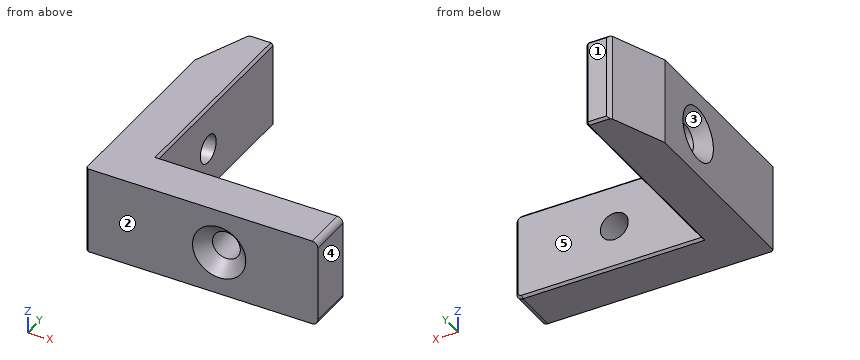
from build123d import *
from OCP.BRepFilletAPI import BRepFilletAPI_MakeChamfer

# Parameters (mm, degrees)
BOSS_EXTRUDE1_DEPTH                                  = 7.5
CSK_FOR_M4_HEX_SOCKET_COUNTERSUNK_HEAD_S_D           = 4.8
CSK_FOR_M4_HEX_SOCKET_COUNTERSUNK_HEAD_S_CSINK_D     = 9.18
CSK_FOR_M4_HEX_SOCKET_COUNTERSUNK_HEAD_S_CSINK_ANGLE = 90
CSK_FOR_M4_HEX_SOCKET_COUNTERSUNK_HE_2_D             = 4.8
CSK_FOR_M4_HEX_SOCKET_COUNTERSUNK_HE_2_CSINK_D       = 9.18
CSK_FOR_M4_HEX_SOCKET_COUNTERSUNK_HE_2_CSINK_ANGLE   = 90
FILLET1_R                                            = 1
CHAMFER1_SIZE                                        = 0.4
CHAMFER1_SIZE2                                       = 0.718021974


with BuildPart() as part:
    # Sketch1 → Boss-Extrude1 (new, symmetric)
    with BuildSketch(Plane.XY):
        Polygon((0, 0), (0, 33), (4, 43), (8, 43), (8, 8), (40, 8), (40, 0), align=None)
    extrude(amount=BOSS_EXTRUDE1_DEPTH, both=True)

    # CSK for M4 Hex Socket Countersunk Head S (through all)
    with Locations(Plane(origin=(0, 0, 0), x_dir=(-1, 0, 0), z_dir=(0, -1, 0))):
        with Locations((-23, 0)):
            CounterSinkHole(CSK_FOR_M4_HEX_SOCKET_COUNTERSUNK_HEAD_S_D / 2, CSK_FOR_M4_HEX_SOCKET_COUNTERSUNK_HEAD_S_CSINK_D / 2, counter_sink_angle=CSK_FOR_M4_HEX_SOCKET_COUNTERSUNK_HEAD_S_CSINK_ANGLE)

    # CSK for M4 Hex Socket Countersunk He 2 (through all)
    with Locations(Plane.ZY):
        with Locations((0, 23)):
            CounterSinkHole(CSK_FOR_M4_HEX_SOCKET_COUNTERSUNK_HE_2_D / 2, CSK_FOR_M4_HEX_SOCKET_COUNTERSUNK_HE_2_CSINK_D / 2, counter_sink_angle=CSK_FOR_M4_HEX_SOCKET_COUNTERSUNK_HE_2_CSINK_ANGLE)

    # Fillet1
    fillet1_edges = [part.edges().sort_by_distance(p)[0] for p in [
        (40, 4, 7.5),
        (40, 4, -7.5),
    ]]
    fillet(fillet1_edges, radius=FILLET1_R)

    # Chamfer1: one chamfer whose edges measure the first distance from different faces: ONE call of the kernel's chamfer builder (chamfer() names one face for all edges)
    chamfer1_edges_1 = [part.edges().sort_by_distance(p)[0] for p in [
        (0, 0, 0),
        (8, 43, 0),
        (8, 25.5, 7.5),
        (6, 43, 7.5),
        (40, 8, 0),
        (23.5, 8, -7.5),
        (23.5, 8, 7.5),
        (39.707106781, 8, 7.207106781),
        (39.707106781, 8, -7.207106781),
        (6, 43, -7.5),
        (8, 25.5, -7.5),
    ]]
    chamfer1_edges_2 = [part.edges().sort_by_distance(p)[0] for p in [
        (4, 43, 0),
    ]]
    chamfer1_side_2 = [part.faces().sort_by_distance(p)[0] for p in [
        (6, 43, 0),
    ]]
    chamfer1 = BRepFilletAPI_MakeChamfer(part.part.solid().wrapped)
    for e in chamfer1_edges_1:
        chamfer1.Add(CHAMFER1_SIZE, e.wrapped)
    for e in chamfer1_edges_2:
        chamfer1.Add(CHAMFER1_SIZE, CHAMFER1_SIZE2, e.wrapped, chamfer1_side_2[0].wrapped)  # the first distance lies on this face
    add(Compound.cast(chamfer1.Shape()), mode=Mode.REPLACE)


solid = part.part
Could you check a few things on this model? Use its own coordinates, in mm. Face numbers are marked on the shaded views. A direction names the side the tool comes from. Round coordinates to 2 decimals unless told otherwise and drop trailing zeros. Write each loop counter-clockwise with the first axis right and the second up, starting at its lowest first coordinate (ties: lowest second). Pieces come first, ordered by that corner, then holes. Notation, with made-up numbers: (89.25, -3.5) - (148.25, -3.5) arc R14 ccw to (148.25, 21.5) - close; hole circle Ø6 at (62.25, -40). An arc over 180 degrees is marked (long way). Put each result on its own line as item: value. Start each with the question number.
(1) I want a section at B-B, the plane z = 0. Please give me the cut outline in (x, y), plus the area to 3 significant figures.
(2) Will these pins go through, and if not, where does the flat tip stop? pin 1 (3 mm diameter, centred on x = 26.5, z = 2, fed in from -Y); pin 2 (6 mm diameter, centred on y = 23, z = 0, fed in from +X); pin 3 (7.5 mm diameter, centred on x = 23, z = 0, fed in from -Y).
(3) Thinking about a two-plate mould opening in Y: for the marked faces 1, 2 and 3, which applies, released by +Y, released by -Y, zero draft, split by the parting line, or undercut?
(4) For the marked faces 4 and 5, which set-ups out of +Z, -Z, +X, -X, +Y, -Y let a thin tool reach every point of the face, with its end or its side?
(5) I want a section at D-D, the plane y = 37.5. Please give me the cut outline in (x, z), plus the area to 3 significant figures.
(6) I want a section at A-A, the plane x = 23. Please give me the cut outline in (y, z).
(7) I need wall thicknesses on probe 1 along Y at (x, z) = (5.4, 0); probe 2 along Z at (x, y) = (23, 6.15); probe 3 along X at (y, z) = (9.5, -3). Which ranges of each line are inside material? Lowest first, please.
Here are the results:
1. outline: (0, 0.4) - (0.4, 0) - (18.41, 0) - (20.6, 2.19) - (20.6, 8) - (8, 8) - (8, 20.6) - (2.19, 20.6) - (0, 18.41) - close; (0, 27.59) - (2.19, 25.4) - (8, 25.4) - (8, 42.6) - (7.6, 43) - (4.4, 43) - (3.73, 42.33) - (0, 33) - close; (25.4, 2.19) - (27.59, 0) - (40, 0) - (40, 7.6) - (39.6, 8) - (25.4, 8) - close
1. area: 493 mm^2
2. pin 1: stops at y = 0
2. pin 2: stops at x = 8
2. pin 3: stops at y = 0.84
3. face 1: released by +Y
3. face 2: released by -Y
3. face 3: undercut
4. face 4: +Z, -Z, +X, +Y, -Y
4. face 5: +Z, -Z, +X, +Y
5. outline: (1.8, -7.5) - (7.6, -7.5) - (8, -7.1) - (8, 7.1) - (7.6, 7.5) - (1.8, 7.5) - close
5. area: 92.8 mm^2
6. outline: (0, -7.5) - (7.6, -7.5) - (8, -7.1) - (8, -2.4) - (2.19, -2.4) - (0, -4.59) - close; (0, 4.59) - (2.19, 2.4) - (8, 2.4) - (8, 7.1) - (7.6, 7.5) - (0, 7.5) - close
7. probe 1: y = 0 to 20.6, 25.4 to 43
7. probe 2: z = -7.5 to -2.4, 2.4 to 7.5
7. probe 3: x = 0 to 8
